The listing builds one solid part. Answer for the finished solid, in the listing's coordinates (mm). Coordinates: 2 decimals unless noted, no trailing zeros. Write each loop counter-clockwise with the first axis right and the second up, starting at its lowest first coordinate (ties: lowest second). Pieces come first, ordered by that corner, then holes. Notation, with made-up numbers: M 67,33.25 L 75,33.25 A29 cw 75,72.25 Z; hole C 67,54 d7. An arc over 180 degrees is marked long. Answer as CSV lines item,"result". Start each with the question number.
```python
from build123d import *

# Parameters (mm, degrees)
SKETCH_1_W      = 9.9
SKETCH_1_H      = 9.9
SKETCH_1_R      = 2.5
EXTRUDE_1_DEPTH = 4
EXTRUDE_2_DEPTH = 4
SKETCH_3_W      = 9.9
SKETCH_3_H      = 9.9
SKETCH_3_R      = 2.5
EXTRUDE_3_DEPTH = 4


with BuildPart() as part:
    # 草图1 → 凸台-拉伸1 (new body)
    with BuildSketch(Plane(origin=(0, 0, 0), x_dir=(1, 0, 0), z_dir=(0, 1, 0))):
        Rectangle(SKETCH_1_W, SKETCH_1_H)
        with Locations(Location((0, 0, 0), (0, 0, 270))):
            Circle(SKETCH_1_R, mode=Mode.SUBTRACT)
    extrude(amount=EXTRUDE_1_DEPTH)

    # 草图2 → 凸台-拉伸2 (add)
    with BuildSketch(Plane(origin=(0, 0, 0), x_dir=(1, 0, 0), z_dir=(0, 1, 0))):
        with BuildLine():
            Line((3.05, -6.95), (-2.95, -6.95))
            ThreePointArc((-2.95, -6.95), (-4.364213562, -6.364213562), (-4.95, -4.95))
            Line((-4.95, -4.95), (-2.95, -4.95))
            ThreePointArc((-2.95, -4.95), (-3.45, -5.45), (-2.95, -5.95))
            Line((-2.95, -5.95), (3.05, -5.95))
            ThreePointArc((3.05, -5.95), (4.8, -7.7), (3.05, -9.45))
            Line((3.05, -9.45), (-2.95, -9.45))
            ThreePointArc((-2.95, -9.45), (-3.7, -10.2), (-2.95, -10.95))
            Line((-2.95, -10.95), (3.05, -10.95))
            ThreePointArc((3.05, -10.95), (4.8, -12.7), (3.05, -14.45))
            Line((3.05, -14.45), (-2.95, -14.45))
            ThreePointArc((-2.95, -14.45), (-3.7, -15.2), (-2.95, -15.95))
            Line((-2.95, -15.95), (3.05, -15.95))
            ThreePointArc((3.05, -15.95), (4.8, -17.7), (3.05, -19.45))
            Line((3.05, -19.45), (-2.95, -19.45))
            ThreePointArc((-2.95, -19.45), (-3.7, -20.2), (-2.95, -20.95))
            Line((-2.95, -20.95), (3.05, -20.95))
            ThreePointArc((3.05, -20.95), (4.8, -22.7), (3.05, -24.45))
            Line((3.05, -24.45), (-2.95, -24.45))
            ThreePointArc((-2.95, -24.45), (-3.7, -25.2), (-2.95, -25.95))
            Line((-2.95, -25.95), (3.05, -25.95))
            ThreePointArc((3.05, -25.95), (4.8, -27.7), (3.05, -29.45))
            Line((3.05, -29.45), (-2.95, -29.45))
            ThreePointArc((-2.95, -29.45), (-3.7, -30.2), (-2.95, -30.95))
            Line((-2.95, -30.95), (3.05, -30.95))
            ThreePointArc((3.05, -30.95), (4.464213562, -31.535786438), (5.05, -32.95))
            Line((5.05, -32.95), (3.05, -32.95))
            ThreePointArc((3.05, -32.95), (3.55, -32.45), (3.05, -31.95))
            Line((3.05, -31.95), (-2.95, -31.95))
            ThreePointArc((-2.95, -31.95), (-4.7, -30.2), (-2.95, -28.45))
            Line((-2.95, -28.45), (3.05, -28.45))
            ThreePointArc((3.05, -28.45), (3.8, -27.7), (3.05, -26.95))
            Line((3.05, -26.95), (-2.95, -26.95))
            ThreePointArc((-2.95, -26.95), (-4.7, -25.2), (-2.95, -23.45))
            Line((-2.95, -23.45), (3.05, -23.45))
            ThreePointArc((3.05, -23.45), (3.8, -22.7), (3.05, -21.95))
            Line((3.05, -21.95), (-2.95, -21.95))
            ThreePointArc((-2.95, -21.95), (-4.7, -20.2), (-2.95, -18.45))
            Line((-2.95, -18.45), (3.05, -18.45))
            ThreePointArc((3.05, -18.45), (3.8, -17.7), (3.05, -16.95))
            Line((3.05, -16.95), (-2.95, -16.95))
            ThreePointArc((-2.95, -16.95), (-4.7, -15.2), (-2.95, -13.45))
            Line((-2.95, -13.45), (3.05, -13.45))
            ThreePointArc((3.05, -13.45), (3.8, -12.7), (3.05, -11.95))
            Line((3.05, -11.95), (-2.95, -11.95))
            ThreePointArc((-2.95, -11.95), (-4.7, -10.2), (-2.95, -8.45))
            Line((-2.95, -8.45), (3.05, -8.45))
            ThreePointArc((3.05, -8.45), (3.8, -7.7), (3.05, -6.95))
        make_face()
    extrude(amount=EXTRUDE_2_DEPTH)

    # 草图3 → 凸台-拉伸3 (add)
    with BuildSketch(Plane(origin=(0, 0, 0), x_dir=(1, 0, 0), z_dir=(0, 1, 0))):
        with Locations((0.1, -37.9)):
            Rectangle(SKETCH_3_W, SKETCH_3_H)
        with Locations(Location((0.1, -37.9, 0), (0, 0, 270))):
            Circle(SKETCH_3_R, mode=Mode.SUBTRACT)
    extrude(amount=EXTRUDE_3_DEPTH)


solid = part.part
```
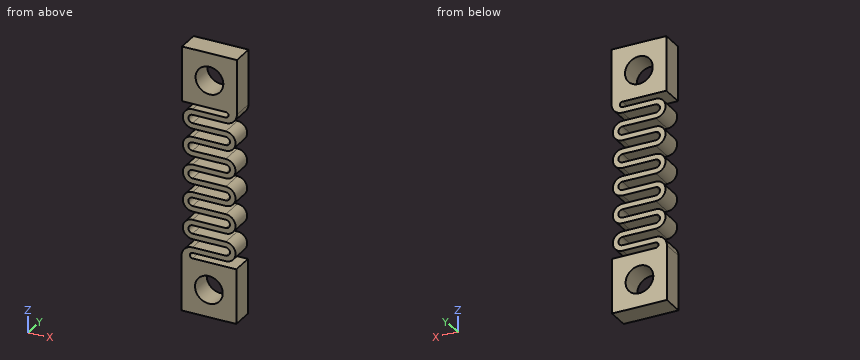
1) The part is cut by section B-B (z = -1.5). Determine the outline of the cut face in (x, y).
2) The part is cut by section D-D (z = 20.2). Determine the outline of the cut face in (x, y), then the cut area to 3 significant figures.
3) Find the intervals of material crossed by line 1 (X direction, y = 1.55, z = 37.9); line 2 (X direction, y = 1.3, z = 0); line 3 (X direction, y = 3.6, z = 30), in increasing order. Write a range as from..to.
4) The part is cut by section C-C (y = 1.85). Count the separate pieces of the cut face and the enclosed holes in it, then the cut area to 3 significant figures.
5) Each of these flat-tipped pins is pushed along its axis until it touches: P1, Ø1.2, axis at y = 1.5, z = 39, coming from the -X side; P2, Ø1.2, axis at y = 2, z = 0, coming from the +X side; P3, Ø4.5, axis at x = 0.1, z = 37.9, coming from the +Y side. Where does it stop, or does it pass through?
6) The part is cut by section A-A (z = 37.9). Determine the outline of the cut face in (x, y).
Completed:
1,outline,"M -4.95,0 L -2,0 L -2,4 L -4.95,4 Z; M 2,0 L 4.95,0 L 4.95,4 L 2,4 Z"
2,outline,"M -4.7,0 L -3.7,0 L -3.7,4 L -4.7,4 Z"
2,area,"4.00 mm²"
3,line 1,"-4.85..-2.4, 2.6..5.05"
3,line 2,"-4.95..-2.5, 2.5..4.95"
3,line 3,"-4.69..-3.67"
4,separate pieces,"1"
4,enclosed holes,"2"
4,area,"268 mm²"
5,P1,"x = -4.85"
5,P2,"x = 4.95"
5,P3,"through"
6,outline,"M -4.85,0 L -2.4,0 L -2.4,4 L -4.85,4 Z; M 2.6,0 L 5.05,0 L 5.05,4 L 2.6,4 Z"
